from build123d import *

# Parameters (mm, degrees)
SKETCH_1_R                = 115
SKETCH_1_R_2              = 105
EXTRUDE_1_DEPTH           = 5
SKETCH_4_R                = 2.5
CUT_EXTRUDE_1_DEPTH       = 33.934862746
EXTRUDE_2_DEPTH           = 5
HOLE_WIZARD_1_D           = 4.5
HOLE_WIZARD_1_CBORE_D     = 6
HOLE_WIZARD_1_CBORE_DEPTH = 3
SKETCH_9_R                = 2.25
SKETCH_9_R_2              = 1.9
EXTRUDE_3_DEPTH           = 5
EXTRUDE_4_DEPTH           = 5
HOLE_WIZARD_2_D           = 4.5
HOLE_WIZARD_2_CBORE_D     = 6
HOLE_WIZARD_2_CBORE_DEPTH = 3
SKETCH_13_R               = 2.25
SKETCH_13_R_2             = 1.9
EXTRUDE_5_DEPTH           = 5
SKETCH_14_W               = 562.038590931
SKETCH_14_H               = 462.09177453
CUT_EXTRUDE_4_DEPTH       = 163.29776757
SKETCH_15_W               = 480.927145246
SKETCH_15_H               = 274.608213656
CUT_EXTRUDE_5_DEPTH       = 161


with BuildPart() as part:
    # 草图1 → 凸台-拉伸1 (new body, symmetric)
    with BuildSketch(Plane.XY):
        Circle(SKETCH_1_R)
        Circle(SKETCH_1_R_2, mode=Mode.SUBTRACT)
    extrude(amount=EXTRUDE_1_DEPTH, both=True)

    # 扫描1: sweep along a path in 草图2
    with BuildLine(Plane(origin=(0, 0, 0), x_dir=(1, 0, 0), z_dir=(0, 1, 0))) as sweep_1_path:
        Line((-130, -355), (-156.694693778, -281.656931626))
        ThreePointArc((-156.694693778, -281.656931626), (-157.1458451, -279.97321197), (-157.29776757, -278.236730193))
        Line((-157.29776757, -278.236730193), (-157.29776757, -10))
        ThreePointArc((-157.29776757, -10), (-154.368835382, -2.928932188), (-147.29776757, 0))
        Line((-147.29776757, 0), (-115, 0))
        Line((-115, 0), (-106.681302201, 0))
    # 草图3 → 扫描1 (sweep)
    with BuildSketch(Plane(origin=(-130, 0, 355), x_dir=(0.939692621, 0, -0.342020143), z_dir=(0.342020143, 0, 0.939692621))):
        Polygon((-5, -15), (5, -15), (5, -11.5), (2, -11.5), (2, 11.5), (5, 11.5), (5, 15), (-5, 15), align=None)
    sweep_1 = sweep(path=sweep_1_path.line)

    # 草图4 → 切除-拉伸1 (cut, through all)
    with BuildSketch(Plane(origin=(-227.008304281, 0, 82.624265689), x_dir=(-0.342020143, 0, -0.939692621), z_dir=(0.939692621, 0, -0.342020143))):
        with Locations((-274.128261747, 6.75)):
            Circle(SKETCH_4_R)
        with Locations((-274.128261747, -6.75)):
            Circle(SKETCH_4_R)
    cut_extrude_1 = extrude(amount=-CUT_EXTRUDE_1_DEPTH, mode=Mode.SUBTRACT)

    # 镜向1: 扫描1, 切除-拉伸1 across plane
    add(sweep_1.mirror(Plane(origin=(0, 0, 0), x_dir=(0, 0, 1), z_dir=(1, 0, 0))))
    add(cut_extrude_1.mirror(Plane(origin=(0, 0, 0), x_dir=(0, 0, 1), z_dir=(1, 0, 0))), mode=Mode.SUBTRACT)

    # 草图6 → 凸台-拉伸2 (add, symmetric)
    with BuildSketch(Plane(origin=(0, 0, 0), x_dir=(0, 0, -1), z_dir=(1, 0, 0))):
        with BuildLine():
            Line((-5, 115), (-5, 125))
            ThreePointArc((-5, 125), (0, 130), (5, 125))
            Line((5, 125), (5, 115))
            Line((5, 115), (5, 112.136445143))
            Line((5, 112.136445143), (-5, 112.136445143))
            Line((-5, 112.136445143), (-5, 115))
        make_face()
    extrude_2 = extrude(amount=EXTRUDE_2_DEPTH, both=True)

    # 镜向2: 凸台-拉伸2 across plane
    add(extrude_2.mirror(Plane.ZX))

    # 孔1 (through all)
    with Locations(Plane(origin=(5, 0, 0), x_dir=(0, 0, -1), z_dir=(1, 0, 0))):
        with Locations((0, 124.156343107), (0, -125)):
            CounterBoreHole(HOLE_WIZARD_1_D / 2, HOLE_WIZARD_1_CBORE_D / 2, HOLE_WIZARD_1_CBORE_DEPTH)

    # 草图9 → 凸台-拉伸3 (add)
    with BuildSketch(Plane.ZY.offset(5)):
        with Locations((0, 124.156343107)):
            Circle(SKETCH_9_R)
        with Locations((0, 124.156343107)):
            Circle(SKETCH_9_R_2, mode=Mode.SUBTRACT)
        with Locations((0, -125)):
            Circle(SKETCH_9_R)
        with Locations((0, -125)):
            Circle(SKETCH_9_R_2, mode=Mode.SUBTRACT)
    extrude(amount=-EXTRUDE_3_DEPTH)

    # 草图10 → 凸台-拉伸4 (add, symmetric)
    with BuildSketch(Plane.XY.offset(155)):
        with BuildLine():
            Line((-162.29776757, 15), (-152.29776757, 15))
            Line((-152.29776757, 15), (-152.29776757, 20))
            ThreePointArc((-152.29776757, 20), (-157.29776757, 25), (-162.29776757, 20))
            Line((-162.29776757, 20), (-162.29776757, 15))
        make_face()
        with BuildLine():
            Line((-152.29776757, -15), (-152.29776757, -20))
            ThreePointArc((-152.29776757, -20), (-157.29776757, -25), (-162.29776757, -20))
            Line((-162.29776757, -20), (-162.29776757, -15))
            Line((-162.29776757, -15), (-152.29776757, -15))
        make_face()
        with BuildLine():
            Line((162.29776757, -15), (152.29776757, -15))
            Line((152.29776757, -15), (152.29776757, -20))
            ThreePointArc((152.29776757, -20), (157.29776757, -25), (162.29776757, -20))
            Line((162.29776757, -20), (162.29776757, -15))
        make_face()
        with BuildLine():
            Line((152.29776757, 15), (152.29776757, 20))
            ThreePointArc((152.29776757, 20), (157.29776757, 25), (162.29776757, 20))
            Line((162.29776757, 20), (162.29776757, 15))
            Line((162.29776757, 15), (152.29776757, 15))
        make_face()
    extrude(amount=EXTRUDE_4_DEPTH, both=True)

    # 孔2 (through all)
    with Locations(Plane.XY.offset(160)):
        with Locations((-157.29776757, 20), (-157.29776757, -20), (157.29776757, 20), (157.29776757, -20)):
            CounterBoreHole(HOLE_WIZARD_2_D / 2, HOLE_WIZARD_2_CBORE_D / 2, HOLE_WIZARD_2_CBORE_DEPTH)

    # 草图13 → 凸台-拉伸5 (add)
    with BuildSketch(Plane(origin=(0, 0, 150), x_dir=(-1, 0, 0), z_dir=(0, 0, -1))):
        with Locations((-157.29776757, 20)):
            Circle(SKETCH_13_R)
        with Locations((-157.29776757, 20)):
            Circle(SKETCH_13_R_2, mode=Mode.SUBTRACT)
        with Locations((-157.29776757, -20)):
            Circle(SKETCH_13_R)
        with Locations((-157.29776757, -20)):
            Circle(SKETCH_13_R_2, mode=Mode.SUBTRACT)
        with Locations((157.29776757, -20)):
            Circle(SKETCH_13_R)
        with Locations((157.29776757, -20)):
            Circle(SKETCH_13_R_2, mode=Mode.SUBTRACT)
        with Locations((157.29776757, 20)):
            Circle(SKETCH_13_R)
        with Locations((157.29776757, 20)):
            Circle(SKETCH_13_R_2, mode=Mode.SUBTRACT)
    extrude(amount=-EXTRUDE_5_DEPTH)

    # 草图14 → 切除-拉伸4 (cut, through all)
    with BuildSketch(Plane(origin=(0, 0, 0), x_dir=(0, 0, -1), z_dir=(1, 0, 0))):
        with Locations((-153.139864812, -31.152254463)):
            Rectangle(SKETCH_14_W, SKETCH_14_H)
    extrude(amount=-CUT_EXTRUDE_4_DEPTH, mode=Mode.SUBTRACT)

    # 草图15 → 切除-拉伸5 (cut, through all)
    with BuildSketch(Plane.XY.offset(155)):
        Rectangle(SKETCH_15_W, SKETCH_15_H)
    extrude(amount=-CUT_EXTRUDE_5_DEPTH, mode=Mode.SUBTRACT)


solid = part.part
The listing builds one solid part. Answer for the finished solid, in the listing's coordinates (mm). A direction names the side the tool comes from. Give positions to 0.01 mm unless a question says otherwise; leave off trailing zeros. Write each loop counter-clockwise with the first axis right and the second up, starting at its lowest first coordinate (ties: lowest second). Pieces come first, ordered by that corner, then holes. Notation, with made-up numbers: (50, 35.25) - (56, 35.25) arc R28 cw to (56, 54.25) - close; hole circle Ø7 at (21.25, 3). An arc over 180 degrees is marked (long way). Use a Markdown table: item, result.
1. For a pull along Z with two mould halves and no side action, classify faces 6 (the cylindrical face through (137.31, 7.5, 339.16)), 7 (the flat face through (158, 0, 155)), 8 (the flat face through (152.298, 14, 216)) as released by +Z, released by -Z, zero draft, split by the parting line, or undercut.
Values follow:
| item | result |
|---|---|
| face 6 | undercut |
| face 7 | released by -Z |
| face 8 | zero draft |
2. Section A-A on y = -2 is taken. Write down the section's boundary in (x, z).
Values follow:
| item | result |
|---|---|
| outline | (128.12, 354.32) - (154.82, 280.97) arc R8 cw to (155.3, 278.24) - (155.3, 155) - (162.3, 155) - (162.3, 278.24) arc R15 ccw to (161.39, 283.37) - (134.7, 356.71) - close |
3. A tool of negligible diameter and unlimited length cuts with its end or side. For faces 1 (the flat face through (160, 20, 157)), 2 (the flat face through (141.655, -0.161, 317.131)), 3 (the flat face through (157.4, 16.7, 160)), 4 (the flat face through (153, -15, 260)), 5 (the flat face through (162.298, 0, 216)), from which of +Z, -Z, +X, -X, +Y, -Y can it reach the whole face along a straight path? Write none if from no direction.
Values follow:
| item | result |
|---|---|
| face 1 | +Z |
| face 2 | -Z, -X |
| face 3 | +Z, +X, -X, +Y |
| face 4 | +Z, +X, -X, -Y |
| face 5 | +Z, -Z, +X, +Y, -Y |
4. Each of these flat-tipped pins is pushed along its axis until it touches: P1, Ø4, axis at y = 15, z = 244, coming from the -X side; P2, Ø3.5, axis at x = 157.3, y = 20, coming from the -Z side; P3, Ø10, axis at y = -17.5, z = 279.5, coming from the -X side; P4, Ø7, axis at y = -1, z = 222.5, coming from the -X side. Where does it stop, or does it pass through?
Values follow:
| item | result |
|---|---|
| P1 | stops at x = 152.3 |
| P2 | passes through |
| P3 | stops at x = 150.58 |
| P4 | stops at x = 155.3 |
5. Find the intervals of material crossed by probe 1 along X at (y, z) = (8, 214); probe 2 along Y at (x, z) = (158, 187.5); probe 3 along X at (y, z) = (0.5, 310.5), in increasing order. Write a range as from..to.
Values follow:
| item | result |
|---|---|
| probe 1 | x = 155.3..162.3 |
| probe 2 | y = -15..15 |
| probe 3 | x = 144.07..151.52 |
